Source: three-view drawing plus pictorial views. Frame: mm from the lowest corner of the part. A direction names the side the tool comes from. Round coordinates to 2 decimals unless told otherwise and drop trailing zeros. Loops run counter-clockwise (first coordinate to the right, second up) from the corner with the lowest first, then second, coordinate; pieces in that order, holes last. Notation, with made-up numbers: (-4.75, 26.5) -> (35.25, 26.5) arc R22 cw to (35.25, 63.5) -> close; hole circle Ø9 at (-2, 77). An arc over 180 degrees is marked (long way). Answer as a JSON object with one key per item and string values. Group by question number.
Item 1: Draft query along Z for the marked faces 3, 4 and 5. Return one class per face: released by +Z, released by -Z, zero draft, split by the parting line, or undercut.
Item 2: Set-up query: the marked faces 1 and 2. Return all of +Z, -Z, +X, -X, +Y, -Y with unobstructed straight access to the full face (end or side cutting, diameter ignored); none if empty.
Item 3: Material intervals for line 1 (Y direction, x = 14.6, z = 11); line 2 (Z direction, x = 4.5, y = 11); line 3 (X direction, y = 5.5, z = 15.75), sorted ascending. Write a range as [from, to].
Item 4: Section query D-D on z = 2.5. Return loops of the section in (x, y), and give its area (3 significant figures).
Item 5: Section query C-C on x = 2.5. Return loops of the section in (y, z).
Item 6: Pin query (flat end, axial travel): pin 1 (0.5 mm diameter, centred on y = 11.5, z = 6.5, fed in from -X); pin 2 (6 mm diameter, centred on x = 5, z = 15.5, fed in from +Y); pin 3 (0.7 mm diameter, centred on x = 2.5, z = 7, fed in from -Y). Return the tip coordinate at first contact, or that it passes through.
Item 7: Section query A-A on y = 11. Return loops of the section in (x, z), and give its area (4 significant figures).
Item 8: Section query B-B on z = 11. Return loops of the section in (x, y), and give its area (4 significant figures).
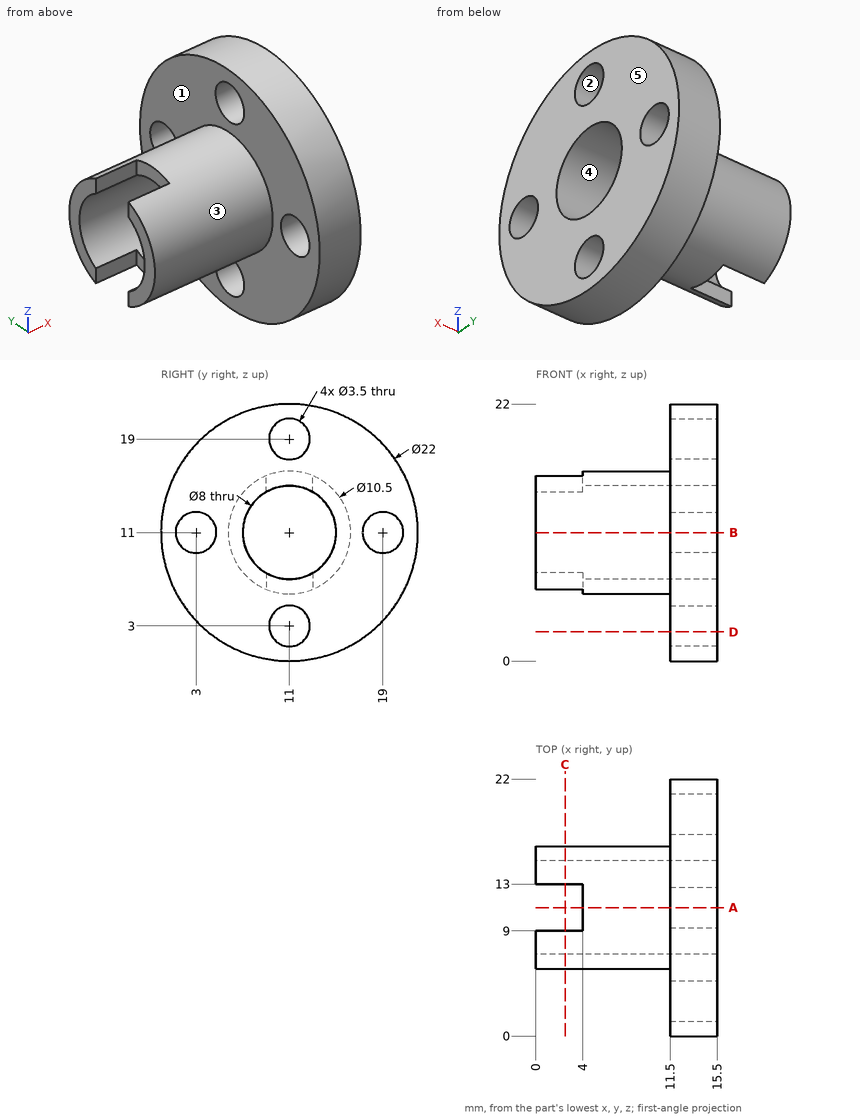
Solved:
{
 "1": {"face 3": "split by the parting line", "face 4": "undercut", "face 5": "zero draft"},
 "2": {"face 1": "-X", "face 2": "+X, -X"},
 "3": {"line 1": "[0, 1.25], [4.75, 7], [15, 17.25], [20.75, 22]", "line 2": "[5.75, 7], [15, 16.25]", "line 3": "[11.5, 15.5]"},
 "4": {"outline": "(11.5, 4.02) -> (15.5, 4.02) -> (15.5, 9.32) -> (11.5, 9.32) -> close; (11.5, 12.68) -> (15.5, 12.68) -> (15.5, 17.98) -> (11.5, 17.98) -> close", "area": "42.4 mm²"},
 "5": {"outline": "(9, 6.15) -> (9, 7.54) arc R4 cw to (9, 14.46) -> (9, 15.85) arc R5.25 ccw to start; (13, 6.15) arc R5.25 ccw to (13, 15.85) -> (13, 14.46) arc R4 cw to (13, 7.54) -> close"},
 "6": {"pin 1": "x = 4", "pin 2": "y = 16.03", "pin 3": "y = 7.23"},
 "7": {"outline": "(4, 5.75) -> (11.5, 5.75) -> (11.5, 4.75) -> (15.5, 4.75) -> (15.5, 7) -> (4, 7) -> close; (4, 15) -> (15.5, 15) -> (15.5, 17.25) -> (11.5, 17.25) -> (11.5, 16.25) -> (4, 16.25) -> close; (11.5, 0) -> (15.5, 0) -> (15.5, 1.25) -> (11.5, 1.25) -> close; (11.5, 20.75) -> (15.5, 20.75) -> (15.5, 22) -> (11.5, 22) -> close", "area": "46.75 mm²"},
 "8": {"outline": "(0, 5.75) -> (11.5, 5.75) -> (11.5, 4.75) -> (15.5, 4.75) -> (15.5, 7) -> (0, 7) -> close; (0, 15) -> (15.5, 15) -> (15.5, 17.25) -> (11.5, 17.25) -> (11.5, 16.25) -> (0, 16.25) -> close; (11.5, 0) -> (15.5, 0) -> (15.5, 1.25) -> (11.5, 1.25) -> close; (11.5, 20.75) -> (15.5, 20.75) -> (15.5, 22) -> (11.5, 22) -> close", "area": "56.75 mm²"}
}
